```python
from build123d import *

# Parameters (mm, degrees)
F0_W     = 19.96
F0_H     = 9.779
F1_DEPTH = 7.239
F2_W     = 19.96
F2_H     = 0.381
F3_DEPTH = 4.699


with BuildPart() as f1:
    # F0 (on Front) → F1 (new body)
    with BuildSketch(Plane.XZ):
        Rectangle(F0_W, F0_H)
    extrude(amount=F1_DEPTH)

    # F2 (on face) → F3 (join)
    with BuildSketch(Plane(origin=(0, 0, 0), x_dir=(-1, 0, 0), z_dir=(0, 1, 0))):
        with Locations((0, -5.08)):
            Rectangle(F2_W, F2_H)
    extrude(amount=-F3_DEPTH)


solid = f1.part
```
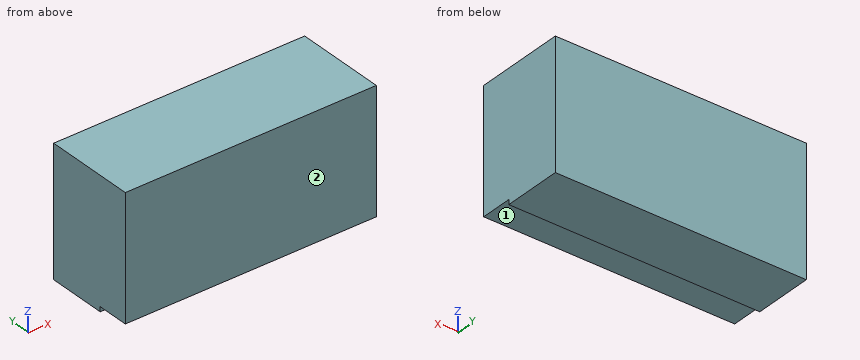
Input: part model. Units: mm. Frame: model coordinates. Face numbers are marked on the shaded views. A direction names the side the tool comes from. Coordinates: 2 decimals unless noted, no trailing zeros. Loops run counter-clockwise (first coordinate to the right, second up) from the corner with the lowest first, then second, coordinate; pieces in that order, holes last. Notation, with made-up numbers: M 58,-12 L 84,-12 A8 cw 84,-4 Z; hole C -10,-25 d6. An arc over 180 degrees is marked long. Use a Markdown table: item, result. Add a question column.
1) Section A-A, the plane y = -5.25. Return the cut outline in (x, z), plus the area to 3 significant figures.
2) Set-up query: the marked faces 1 and 2. Return all of +Z, -Z, +X, -X, +Y, -Y with unobstructed straight access to the full face (end or side cutting, diameter ignored); none if empty.
3) Line query: L1, parallel to Z at x = 7.25, y = -7. Output: solid intervals per line, ascending. Write a range as from..to.
4) Pin query (flat end, axial travel): P1, Ø2, axis at x = 2, y = -5.5, coming from the -Z side. Return the tip coordinate at first contact, or that it passes through.
Answer below:
| question | item | result |
|---|---|---|
| 1 | outline | M -9.98,-4.89 L 9.98,-4.89 L 9.98,4.89 L -9.98,4.89 Z |
| 1 | area | 195 mm2 |
| 2 | face 1 | -Z, +X, -X, -Y |
| 2 | face 2 | +Z, -Z, +X, -X, -Y |
| 3 | L1 | -4.89..4.89 |
| 4 | P1 | z = -5.27 |
